Here's the drawing with two shaded views (mm, measured from the low corner). I have some questions. A direction names the side the tool comes from. Coordinates: 2 decimals unless noted, no trailing zeros. Write each loop counter-clockwise with the first axis right and the second up, starting at its lowest first coordinate (ties: lowest second). Pieces come first, ordered by that corner, then holes.
Item 1: I want a section at B-B on y = 10. Please give me the cut outline in (x, z), then the cut area to 3 significant figures.
Item 2: I want a section at A-A on z = 7. Please give me the cut outline in (x, y).
Item 3: I want a section at C-C on x = 13.5. Please give me the cut outline in (y, z) (3 decimals).
Item 4: I want a section at D-D on z = 14.25. Please give me the cut outline in (x, y) (3 decimals), then the cut area to 3 significant figures.
Item 5: If I drill on probe 1 along X at (y, z) = (9.75, 15.25); probe 2 along X at (y, z) = (14.5, 12.75); probe 3 along Z at (x, y) = (15.5, 6), over which ranges is the centre line in solid material (lowest first)?
Item 6: For P1, Ø3, axis at y = 12, z = 17, coming from the +X side; P2, Ø6, axis at y = 16.5, z = 3, coming from the -X side; P3, Ø1, axis at y = 11.5, z = 16.5, coming from the +X side, each with a flat end and sliding along its axis, tell me the tip position at first contact or that it passes through.
Item 7: Which directions (+Z, -Z, +X, -X, +Y, -Y) give clear straight access to the entire face, cutting with the end or side of a thin tool? Please do the marked faces 1, 2, 3 and 4.
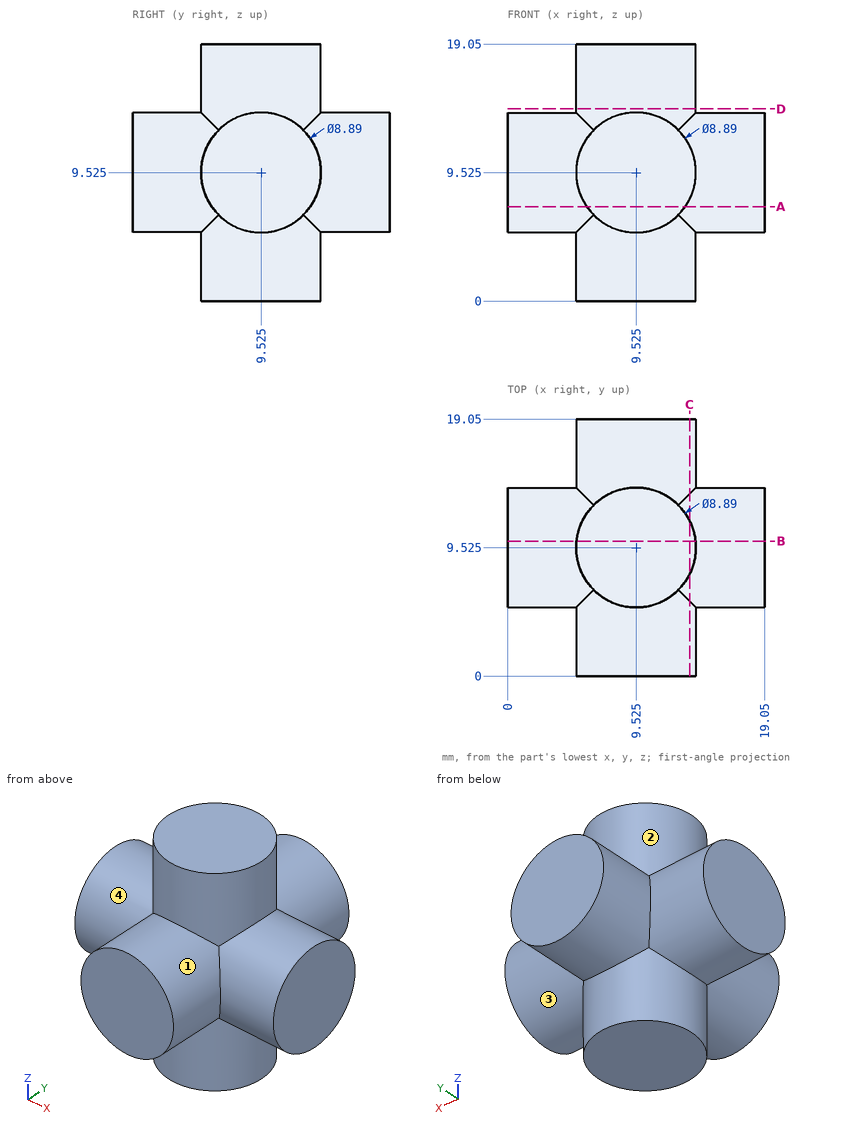
Response values:
1. outline: (0, 5.11) - (5.11, 5.11) - (5.11, 0) - (13.94, 0) - (13.94, 5.11) - (19.05, 5.11) - (19.05, 13.94) - (13.94, 13.94) - (13.94, 19.05) - (5.11, 19.05) - (5.11, 13.94) - (0, 13.94) - close
1. area: 259 mm2
2. outline: (0, 5.87) - (5.87, 5.87) - (5.87, 0) - (13.18, 0) - (13.18, 5.87) - (19.05, 5.87) - (19.05, 13.18) - (13.18, 13.18) - (13.18, 19.05) - (5.87, 19.05) - (5.87, 13.18) - (0, 13.18) - close
3. outline: (0, 7.536) - (5.55, 7.536) arc R4.445 ccw to (7.536, 5.55) - (7.536, 0) - (11.514, 0) - (11.514, 5.55) arc R4.445 ccw to (13.5, 7.536) - (19.05, 7.536) - (19.05, 11.514) - (13.5, 11.514) arc R4.445 ccw to (11.514, 13.5) - (11.514, 19.05) - (7.536, 19.05) - (7.536, 13.5) arc R4.445 ccw to (5.55, 11.514) - (0, 11.514) - close
4. outline: circle Ø8.89 at (9.525, 9.525)
4. area: 62.1 mm2
5. probe 1: x = 5.09 to 13.96
5. probe 2: x = 6.47 to 12.58
5. probe 3: z = 6.82 to 12.23
6. P1: stops at x = 13.86
6. P2: stops at x = 6.82
6. P3: stops at x = 13.72
7. face 1: -Y
7. face 2: +Z
7. face 3: +X
7. face 4: -X
